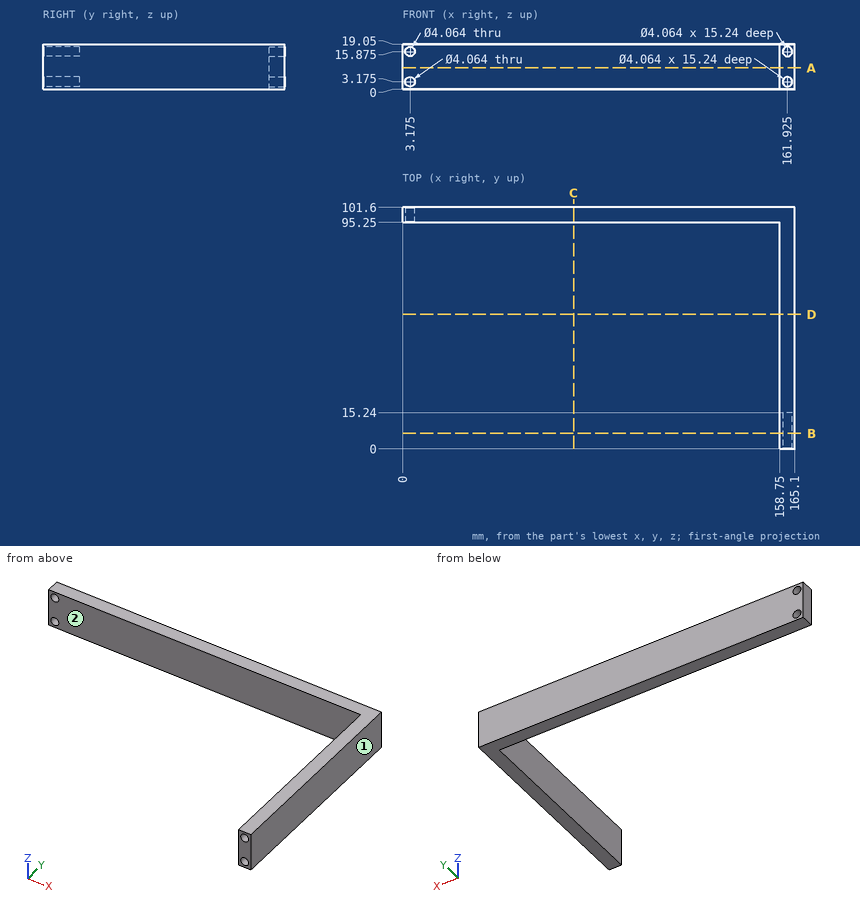
Input: dimensioned drawing with shaded views. Units: mm. Origin: part minimum x, y, z. A direction names the side the tool comes from. Coordinates: 2 decimals unless noted, no trailing zeros. Write each loop counter-clockwise with the first axis right and the second up, starting at its lowest first coordinate (ties: lowest second). Pieces come first, ordered by that corner, then holes. Notation, with made-up numbers: M 52,-18 L 90,-18 A27 ccw 90,12 Z; hole C 20.25,-34 d4. An arc over 180 degrees is marked long. Use one line per item in the form item = value.
Q1. First-contact query: pin 1 (1.2 mm diameter, centred on x = 162, z = 3, fed in from -Y); pin 2 (2 mm diameter, centred on y = 37.5, z = 7, fed in from -X); pin 3 (1 mm diameter, centred on x = 108, z = 10, fed in from -Y); pin 4 (4.5 mm diameter, centred on x = 3.175, z = 15.875, fed in from +Y). Flat tips, straight axial feed; report the tip coordinate or a pass-through.
Answer below:
pin_1 = 15.24
pin_2 = 158.75
pin_3 = 95.25
pin_4 = 101.6
Q2. Material intervals for probe 1 along Y at (x, z) = (145, 15); probe 2 along X at (y, z) = (97.5, 15); probe 3 along X at (y, z) = (27.5, 18), sorted ascending. Write a range as from..to.
Answer below:
probe_1 = 95.25..101.6
probe_2 = 0..1.34, 5.01..165.1
probe_3 = 158.75..165.1
Q3. Section B-B (y = 6.5). Return loops of the section in (x, z) (3 decimals), plus the area to 3 significant figures.
Answer below:
outline = M 158.75,0 L 165.1,0 L 165.1,19.05 L 158.75,19.05 Z; hole C 161.925,3.175 d4.064; hole C 161.925,15.875 d4.064
area = 95.0 mm²
Q4. Set-up query: the marked faces 1 and 2. Return all of +Z, -Z, +X, -X, +Y, -Y with unobstructed straight access to the full face (end or side cutting, diameter ignored); none if empty.
Answer below:
face_1 = +Z, -Z, +X, +Y, -Y
face_2 = +Z, -Z, -X, -Y
Q5. Section C-C (x = 72). Return loops of the section in (y, z), plus the area to 3 significant figures.
Answer below:
outline = M 95.25,0 L 101.6,0 L 101.6,19.05 L 95.25,19.05 Z
area = 121 mm²
Q6. Section A-A (z = 9). Return loops of the section in (x, y).
Answer below:
outline = M 0,95.25 L 158.75,95.25 L 158.75,0 L 165.1,0 L 165.1,101.6 L 0,101.6 Z
Q7. Section D-D (y = 56.5). Return loops of the section in (x, z).
Answer below:
outline = M 158.75,0 L 165.1,0 L 165.1,19.05 L 158.75,19.05 Z
